Input: part model. Units: mm. Frame: model coordinates. A direction names the side the tool comes from. Give positions to 0.01 mm unless a question says otherwise; leave off trailing zeros. Loops run counter-clockwise (first coordinate to the right, second up) from the corner with the lowest first, then second, coordinate; pieces in that order, holes last. Notation, with made-up numbers: M -33.5,-8.5 L 25.5,-8.5 A24 ccw 25.5,11.5 Z; hole C 38.25,-31.5 d11. An arc over 180 degrees is marked long. Answer as a JSON object with one key per item and string values. Group by question number.
1) Section query B-B on z = 0. Return loops of the section in (x, y), plus the area to 3 significant figures.
2) First-contact query: P1, Ø0.5, axis at x = 0, z = -4, coming from the -Y side; P2, Ø0.6, axis at x = -1, z = -5.5, coming from the -Y side. Flat tips, straight axial feed; report the tip coordinate or a pass-through.
3) Draft query along X for faces 1 (the flat face through (-1, 2.65, -5)), 2 (the cylindrical face through (-2.715, -0.246, 7.699)), 3 (the flat face through (-0.3, 0, 5)). Return one class per face: +X half, -X half, draft (parallel to the pull), parting line (faces both ways), or undercut.
4) Section query A-A on y = 1.25. Return loops of the section in (x, z), plus the area to 3 significant figures.
5) Access query for faces 4 (the flat face through (0, 2.4, -5)), 5 (the flat face through (-1, 2.65, 5)), 6 (the flat face through (1, 1.5, -5)). Directions: +Z, -Z, +X, -X, +Y, -Y. A direction counts if a zero-diameter tool reaches every point of the face in a straight line with its end or side. Return the directions, or none.
6) Ray query, L1, parallel to Z at x = 0, y = 0.4; L2, parallel to Z at x = -0.1, y = -0.8; L3, parallel to Z at x = -0.9, y = 0.2. Return the intervals inside material, ascending.
Autodesk Inventor part; units mm, degrees
ref_plane "YZ Plane" through (0, 0, 0) normal (1, 0, 0) x (0, 1, 0)
ref_plane "XZ Plane" through (0, 0, 0) normal (0, 1, 0) x (-1, 0, 0)
ref_plane "XY Plane" through (0, 0, 0) normal (0, 0, 1) x (1, 0, 0)
sketch "Sketch1" plane through (0, 0, 0) normal (0, 1, 0) x (-1, 0, 0)
  line L0 (2, 8) -> (-2, 8)
  line L1 (-3, 7) -> (-3, 3)
  line L2 (-2, -8) -> (2, -8)
  line L3 (3, -7) -> (3, 7)
  circle A0 centre (0, 5) radius 2.4
  circle A1 centre (0, -5) radius 2.4
  arc A2 (3, 7) -> (2, 8) centre (2, 7) ccw
  arc A3 (-2, 8) -> (-3, 7) centre (-2, 7) ccw
  arc A4 (-3, -7) -> (-2, -8) centre (-2, -7) ccw
  arc A5 (2, -8) -> (3, -7) centre (2, -7) ccw
  line L4 (2, 2) -> (2, 2)
  line L5 (2, -2) -> (2, -2)
  line L6 (-2, 2) -> (-2, 2)
  line L7 (-2, -2) -> (-2, -2)
  line L8 (3, 3) -> (3, 7)
  line L9 (-3, 7) -> (-3, 1.5)
  line L10 (-2.5, -1) -> (-1.5, -1)
  line L11 (-1, -0.5) -> (-1, 0.5)
  line L12 (-1.5, 1) -> (-2.5, 1)
  line L13 (-3, -1.5) -> (-3, -7)
  arc A6 (-2.5, -1) -> (-3, -1.5) centre (-2.5, -1.5) ccw
  arc A7 (-3, 1.5) -> (-2.5, 1) centre (-2.5, 1.5) ccw
  arc A8 (-1.5, -1) -> (-1, -0.5) centre (-1.5, -0.5) ccw
  arc A9 (-1, 0.5) -> (-1.5, 1) centre (-1.5, 0.5) ccw
  point P0 (0, 0)
  point P1 (-3, -8)
  point P2 (-3, 8)
  point P3 (3, -8)
  point P4 (1, -2)
  point P5 (1, 2)
  point P6 (3, -2)
  point P7 (-3, 2)
  point P8 (-1, -2)
  point P9 (-3, -2)
  point P10 (-3, -1)
  point P11 (-1, 1)
  point P12 (-1, -1)
  point P13 (-3, 1)
  dimension "d0" = 6
  dimension "d1" = 16
  dimension "d2" = 4.8
  dimension "d3" = 4.8
  dimension "d5" = 3
  dimension "d6" = 1
  dimension "d7" = 2
  dimension "d8" = 4
  dimension "d9" = 2
  dimension "d70" = 2
  dimension "d71" = 2
  dimension "d72" = 0.5
extrude "Extrusion1" add sketch "Sketch1" against normal blind 0.5 contours A2 L3 A5 L2 A4 L13 A6 L10 A8 L11 A9 L12 A7 L9 L1 A3 L0 | A0 | A1
extrude "Extrusion2" add sketch "Sketch1" along normal blind 2.65 contours A0 | A1
fillet "Fillet1" radius 0.5 2 edges at (2.4, 2.65, 5) (2.4, 2.65, -5)
sketch "Sketch2" plane through (0, -0.5, 0) normal (0, -1, 0) x (1, 0, 0)
  circle A0 centre (0, 5) radius 1.5
  circle A1 centre (0, -5) radius 1.5
  circle A2 centre (0, 5) radius 2
  circle A3 centre (0, -5) radius 2
  point P0 (0, 0)
  dimension "d18" = 3
  dimension "d19" = 3
  dimension "d22" = 4
  dimension "d23" = 4
extrude "Extrusion3" cut sketch "Sketch2" against normal blind 2 contours A0 | A1
extrude "Extrusion4" add sketch "Sketch2" along normal blind 0.75
sketch "Sketch4" plane through (0, -0.5, 0) normal (0, -1, 0) x (1, 0, 0)
  line L0 (0.3, 6.75) -> (-0.3, 6.75)
  line L1 (-0.3, 6.75) -> (-0.3, 3.25)
  line L2 (-0.3, 3.25) -> (0.3, 3.25)
  line L3 (0.3, 3.25) -> (0.3, 6.75)
  line L4 (0.3, -3.25) -> (-0.3, -3.25)
  line L5 (-0.3, -3.25) -> (-0.3, -6.75)
  line L6 (-0.3, -6.75) -> (0.3, -6.75)
  line L7 (0.3, -6.75) -> (0.3, -3.25)
  circle A0 centre (0, 5) radius 1.5
  circle A1 centre (0, -5) radius 1.5
  circle A2 centre (0, 5) radius 0.3
  circle A3 centre (0, -5) radius 0.3
  point P0 (0, 0)
  dimension "d26" = 0.6
  dimension "d27" = 3.5
  dimension "d28" = 0.6
  dimension "d29" = 3.5
  dimension "d32" = 1.2
  dimension "d33" = 1.2
  dimension "d34" = 0.6
  dimension "d35" = 0.6
extrude "Extrusion5" add sketch "Sketch4" against normal blind 2 and the other way blind 0.5 contours L3 A0 L1 L0 | L3 A2 L1 A0 | A2 | L3 A0 L1 A2 | A0 L3 L2 L1 | L7 A1 L5 L4 | L7 A3 L5 A1 | A3 | L7 A1 L5 A3 | A1 L7 L6 L5
extrude "Extrusion6" add sketch "Sketch4" along normal blind 0.75 contours A2 | A3
sketch "Sketch6" plane through (0, 2.65, 5) normal (0, 1, 0) x (1, 0, 0)
  line L0 (0.625, 1) -> (0.375, 1)
  line L1 (0.375, 1) -> (0.375, -1)
  line L2 (0.375, -1) -> (0.625, -1)
  line L3 (0.625, -1) -> (0.625, 1)
  line L4 (0.125, -1) -> (0.125, 1)
  line L5 (0.125, 1) -> (-0.125, 1)
  line L6 (-0.125, 1) -> (-0.125, -1)
  line L7 (-0.125, -1) -> (0.125, -1)
  line L8 (-0.375, -1) -> (-0.375, 1)
  line L9 (-0.375, 1) -> (-0.625, 1)
  line L10 (-0.625, 1) -> (-0.625, -1)
  line L11 (-0.625, -1) -> (-0.375, -1)
  point P0 (0, 5)
  point P1 (0, 0)
  dimension "d47" = 0.25
  dimension "d48" = 2
  dimension "d50" = 1
  dimension "d54" = 0.5
  dimension "d59" = 0.625
sketch "Sketch5" plane through (0, 2.65, -5) normal (0, 1, 0) x (1, 0, 0)
  line L0 (-0.8, 0.8) -> (0.2, 0.8)
  line L1 (0.2, -0.8) -> (-0.8, -0.8)
  line L2 (-0.8, -0.8) -> (-0.8, 0.8)
  line L3 (0.2, 0.8) -> (0.2, 1.0087)
  line L4 (0.2, 1.0087) -> (1.0464, 0)
  line L5 (1.0464, 0) -> (0.2, -1.0087)
  line L6 (0.2, -1.0087) -> (0.2, -0.8)
  point P0 (0, -5)
  point P1 (0, 0)
  point P2 (0, 0)
  dimension "d40" = 40
  dimension "d41" = 100
  dimension "d43" = 1.6
  dimension "d44" = 1
  dimension "d62" = 0.8
  dimension "d69" = 0.8
extrude "Extrusion7" cut sketch "Sketch5" against normal blind 0.25
extrude "Extrusion8" cut sketch "Sketch6" against normal blind 0.25
fillet "Fillet6" radius 0.05 7 edges at (-0.8, 2.525, -5.8) (0.2, 2.525, -5.8) (0.2, 2.525, -6.0087) (1.0464, 2.525, -5) (0.2, 2.525, -3.9913) (0.2, 2.525, -4.2) (-0.8, 2.525, -4.2)
fillet "Fillet9" radius 0.05 12 edges at (0.625, 2.525, 6) (0.125, 2.525, 6) (-0.375, 2.525, 6) (0.625, 2.525, 4) (0.125, 2.525, 4) (-0.375, 2.525, 4) (0.375, 2.525, 4) (-0.125, 2.525, 4) (-0.625, 2.525, 4) (0.375, 2.525, 6) (-0.125, 2.525, 6) (-0.625, 2.525, 6)
properties part number "system-buttons"
Output:
{
 "1": {"outline": "M -3,-0.5 L 1,-0.5 L 1,0 L -3,0 Z", "area": "2.00 mm^2"},
 "2": {"P1": "stops at y = -1", "P2": "stops at y = 1.5"},
 "3": {"face 1": "draft", "face 2": "-X half", "face 3": "undercut"},
 "4": {"outline": "C 0,-5 d4.8; C 0,5 d4.8; hole M -0.3,-6.47 L -0.3,-3.53 A1.5 ccw Z; hole M -0.3,3.53 L -0.3,6.47 A1.5 ccw Z; hole M 0.3,-6.47 A1.5 ccw 0.3,-3.53 Z; hole M 0.3,3.53 A1.5 ccw 0.3,6.47 Z", "area": "25.6 mm^2"},
 "5": {"face 4": "+Y", "face 5": "+Z, -Z, +X, -X, +Y", "face 6": "-Y"},
 "6": {"L1": "z = -7.4 to -2.6, 2.6 to 7.4", "L2": "z = -7 to -3, 3 to 7", "L3": "z = -7.22 to -6.2, -3.8 to -2.78, 2.78 to 3.8, 6.2 to 7.22"}
}
